Geometry check sheet. Reference: the model listing, model coordinates, mm. Coordinates: 2 decimals unless noted, no trailing zeros. Order: outer loops, then holes, each group sorted by start corner. A loop starts at its lowest first (then second) coordinate and runs counter-clockwise, first axis right, second up. Notation, with made-up numbers: (22.25, 31) - (31.25, 31) arc R12 cw to (31.25, 43) - close; hole circle Ø3 at (-18.5, 10). An arc over 180 degrees is marked (long way). Use CSV: the item, a comma, the result in double quotes. Start each with the question number.
1) Sectioned sample at B-B, the plane x = 419. Record the cut outline in (y, z).
2) Thickness scan on probe 1 along Z at (x, y) = (203, -1); probe 2 along Z at (x, y) = (165.4, -11.5); probe 3 along X at (y, z) = (-13.25, 47.5). Record the ranges inside material, lowest first. Write a range as [from, to].
3) Sectioned sample at A-A, the plane x = 366. Record the cut outline in (y, z).
4) Depth check by flat-ended pin: P1, Ø3.5, axis at x = 165.4, z = 32, coming from the -Y side; P2, Ø4, axis at x = 111.5, z = 48.5, coming from the +Y side; P3, Ø2.5, axis at x = 440.8, z = 31.5, coming from the +Y side. Enter the tip coordinate at first touch or a pass-through.
from build123d import *

# Parameters (mm, degrees)
SKETCH_W        = 450.8
SKETCH_H        = 64
SKETCH_R        = 1.5
PAD_DEPTH       = 15
POCKET_DEPTH    = 12
POCKET001_DEPTH = 7.5
SKETCH003_R     = 1.5
HOLE_DEPTH      = 7.5
HOLE_TIPS_R     = 1.5


with BuildPart() as part:
    # Sketch → Pad (new body)
    with BuildSketch(Plane.XZ):
        with Locations((225.4, 32)):
            Rectangle(SKETCH_W, SKETCH_H)
        with Locations((165.4, 32)):
            Circle(SKETCH_R, mode=Mode.SUBTRACT)
        with Locations((285.4, 32)):
            Circle(SKETCH_R, mode=Mode.SUBTRACT)
        with BuildLine():
            Line((300.8, 56.5), (398.8, 56.5))
            ThreePointArc((399.8, 55.5), (399.507107, 56.207107), (398.8, 56.5))
            Line((399.8, 55.5), (399.8, 8.5))
            ThreePointArc((398.8, 7.5), (399.507107, 7.792893), (399.8, 8.5))
            Line((398.8, 7.5), (300.8, 7.5))
            ThreePointArc((299.8, 8.5), (300.092893, 7.792893), (300.8, 7.5))
            Line((299.8, 8.5), (299.8, 55.5))
            ThreePointArc((300.8, 56.5), (300.092893, 56.207107), (299.8, 55.5))
        make_face(mode=Mode.SUBTRACT)
    extrude(amount=PAD_DEPTH)

    # Sketch001 (on DatumPlane) → Pocket (cut)
    with BuildSketch(Plane.XZ):
        with BuildLine():
            Line((297.05, 60.25), (402.55, 60.25))
            ThreePointArc((403.55, 59.25), (403.257107, 59.957107), (402.55, 60.25))
            Line((403.55, 59.25), (403.55, 4.75))
            ThreePointArc((402.55, 3.75), (403.257107, 4.042893), (403.55, 4.75))
            Line((402.55, 3.75), (297.05, 3.75))
            ThreePointArc((296.05, 4.75), (296.342893, 4.042893), (297.05, 3.75))
            Line((296.05, 4.75), (296.05, 59.25))
            ThreePointArc((297.05, 60.25), (296.342893, 59.957107), (296.05, 59.25))
        make_face()
    extrude(amount=POCKET_DEPTH, mode=Mode.SUBTRACT)

    # Sketch002 (on DatumPlane) → Pocket001 (cut)
    with BuildSketch(Plane.XZ):
        with BuildLine():
            Line((21, 51.5), (295.05, 51.5))
            ThreePointArc((295.05, 51.5), (295.757107, 51.792893), (296.05, 52.5))
            Line((296.05, 52.5), (403.55, 52.5))
            ThreePointArc((403.55, 52.5), (403.842893, 51.792893), (404.55, 51.5))
            Line((404.55, 51.5), (429.8, 51.5))
            ThreePointArc((430.8, 50.5), (430.507107, 51.207107), (429.8, 51.5))
            Line((430.8, 50.5), (430.8, 37.5))
            ThreePointArc((429.8, 36.5), (430.507107, 36.792893), (430.8, 37.5))
            Line((429.8, 36.5), (404.55, 36.5))
            ThreePointArc((404.55, 36.5), (403.842893, 36.207107), (403.55, 35.5))
            Line((296.05, 35.5), (403.55, 35.5))
            ThreePointArc((296.05, 35.5), (295.757107, 36.207107), (295.05, 36.5))
            Line((295.05, 36.5), (21, 36.5))
            ThreePointArc((20, 37.5), (20.292893, 36.792893), (21, 36.5))
            Line((20, 37.5), (20, 50.5))
            ThreePointArc((21, 51.5), (20.292893, 51.207107), (20, 50.5))
        make_face()
    extrude(amount=POCKET001_DEPTH, mode=Mode.SUBTRACT)

    # Sketch003 (on DatumPlane) → Hole (cut)
    with BuildSketch(Plane.XZ):
        with Locations((10, 56.5)):
            Circle(SKETCH003_R)
        with Locations((10, 31.5)):
            Circle(SKETCH003_R)
        with Locations((10, 10)):
            Circle(SKETCH003_R)
        with Locations((440.8, 56.5)):
            Circle(SKETCH003_R)
        with Locations((440.8, 31.5)):
            Circle(SKETCH003_R)
        with Locations((440.8, 10)):
            Circle(SKETCH003_R)
    extrude(amount=HOLE_DEPTH, mode=Mode.SUBTRACT)

    # Hole tips → Hole tip 1 section 0
    with BuildSketch(Plane.XZ.offset(7.5), mode=Mode.PRIVATE) as hole_tip_1_s0:
        with Locations((10, 56.5)):
            Circle(HOLE_TIPS_R)
    loft([hole_tip_1_s0.sketch, Vertex(10, -8.401291, 56.5)], mode=Mode.SUBTRACT)

    # Hole tips → Hole tip 2 section 0
    with BuildSketch(Plane.XZ.offset(7.5), mode=Mode.PRIVATE) as hole_tip_2_s0:
        with Locations((10, 31.5)):
            Circle(HOLE_TIPS_R)
    loft([hole_tip_2_s0.sketch, Vertex(10, -8.401291, 31.5)], mode=Mode.SUBTRACT)

    # Hole tips → Hole tip 3 section 0
    with BuildSketch(Plane.XZ.offset(7.5), mode=Mode.PRIVATE) as hole_tip_3_s0:
        with Locations((10, 10)):
            Circle(HOLE_TIPS_R)
    loft([hole_tip_3_s0.sketch, Vertex(10, -8.401291, 10)], mode=Mode.SUBTRACT)

    # Hole tips → Hole tip 4 section 0
    with BuildSketch(Plane.XZ.offset(7.5), mode=Mode.PRIVATE) as hole_tip_4_s0:
        with Locations((440.8, 56.5)):
            Circle(HOLE_TIPS_R)
    loft([hole_tip_4_s0.sketch, Vertex(440.8, -8.401291, 56.5)], mode=Mode.SUBTRACT)

    # Hole tips → Hole tip 5 section 0
    with BuildSketch(Plane.XZ.offset(7.5), mode=Mode.PRIVATE) as hole_tip_5_s0:
        with Locations((440.8, 31.5)):
            Circle(HOLE_TIPS_R)
    loft([hole_tip_5_s0.sketch, Vertex(440.8, -8.401291, 31.5)], mode=Mode.SUBTRACT)

    # Hole tips → Hole tip 6 section 0
    with BuildSketch(Plane.XZ.offset(7.5), mode=Mode.PRIVATE) as hole_tip_6_s0:
        with Locations((440.8, 10)):
            Circle(HOLE_TIPS_R)
    loft([hole_tip_6_s0.sketch, Vertex(440.8, -8.401291, 10)], mode=Mode.SUBTRACT)


solid = part.part
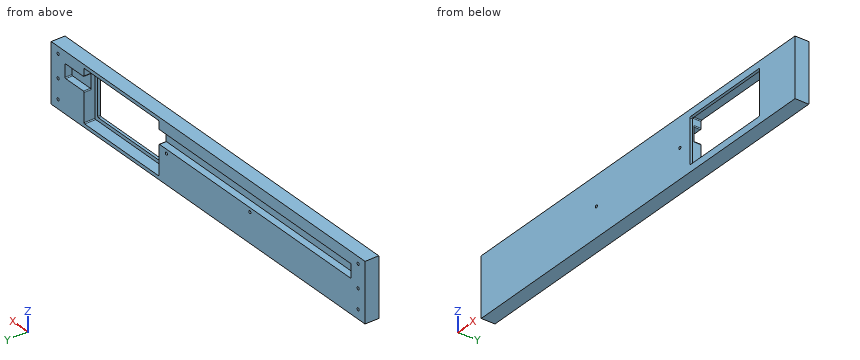
Evaluation:
1,outline,"(-15, 0) - (0, 0) - (0, 36.5) - (-7.5, 36.5) - (-7.5, 51.5) - (0, 51.5) - (0, 64) - (-15, 64) - close"
2,probe 1,"[0, 36.5], [51.5, 64]"
2,probe 2,"[0, 30.5], [33.5, 64]"
2,probe 3,"[0, 299.8], [399.8, 450.8]"
3,outline,"(-15, 0) - (0, 0) - (0, 3.75) - (-12, 3.75) - (-12, 7.5) - (-15, 7.5) - close; (-15, 56.5) - (-12, 56.5) - (-12, 60.25) - (0, 60.25) - (0, 64) - (-15, 64) - close"
4,P1,"y = -15"
4,P2,"y = -7.5"
4,P3,"y = -7.65"
